Part model, mm, in its own coordinate system. Face numbers are marked on the shaded views. A direction names the side the tool comes from. Round coordinates to 2 decimals unless told otherwise and drop trailing zeros. Write each loop counter-clockwise with the first axis right and the second up, starting at its lowest first coordinate (ties: lowest second). Pieces come first, ordered by that corner, then holes. Notation, with made-up numbers: M 3.5,33.25 L 21.5,33.25 A29 cw 21.5,60.25 Z; hole C 72,45 d2. An arc over 180 degrees is marked long. One line per question, with ' | ' between items. Start each with the question number.
1) Saw through at C-C (x = -48). List the corners of the cut face in (y, z).
2) Wall check: probe 1 along Z at (x, y) = (-23, 23.5); probe 2 along Y at (x, z) = (32, 54.5); probe 3 along Y at (x, z) = (18.5, -50.5). Give the ranges that are in metal, low to high. Write a range as [from, to].
3) Saw through at A-A (x = 20). List the corners of the cut face in (y, z), plus the area to 3 significant figures.
4) Tool access for the marked faces 1, 2 and 3: list every direction of +Z, -Z, +X, -X, +Y, -Y with a clear straight run to the whole face (end or side of a thin tool).
5) Saw through at B-B (y = 6.25). List the corners of the cut face in (x, z), plus the area to 3 significant figures.
6) Saw through at D-D (z = -35.5). List the corners of the cut face in (x, y), plus the area to 3 significant figures.
7) Drop flat-ended pins along their axis: pin 1 Ø10 at (x, z) = (-9.5, 10.5) entering from -Y; pin 2 Ø12 at (x, y) = (-20.5, 15) entering from -Z; pin 3 Ø8 at (x, z) = (-27.5, 48) entering from -Y; pin 4 Ø16 at (x, z) = (-19.5, 4) entering from -Y. Give the stop position or say it passes through.
8) Mould opens along X. For the marked faces 4, 5 and 6 say: pulls with the +X half, pulls with the -X half, needs draft (parallel to the pull), parting line crosses it, or undercut.
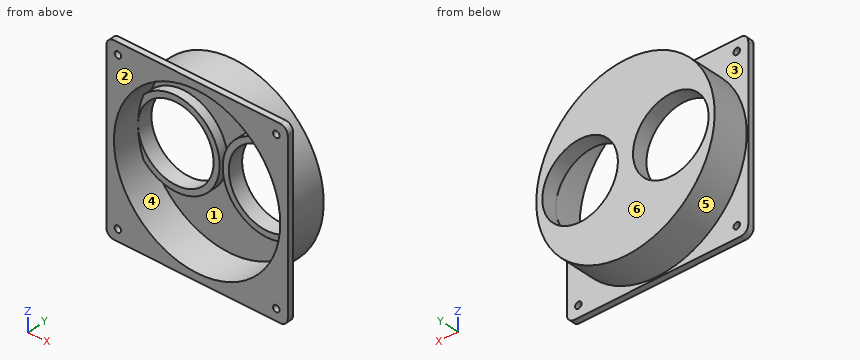
```python
from build123d import *

# Parameters (mm, degrees)
SKETCH1_W           = 120
SKETCH1_H           = 120
BOSS_EXTRUDE1_DEPTH = 4
FILLET1_R           = 5
SKETCH2_R           = 2.15
CUT_EXTRUDE1_DEPTH  = 4
SKETCH3_R           = 55
CUT_EXTRUDE2_DEPTH  = 4
BOSS_EXTRUDE2_START = 20
SKETCH5_R           = 59
SKETCH5_R_2         = 55
BOSS_EXTRUDE2_DEPTH = 20
BOSS_EXTRUDE3_START = 4
SKETCH6_R           = 59
BOSS_EXTRUDE3_DEPTH = 4
SKETCH7_R           = 25
CUT_EXTRUDE3_DEPTH  = 4
SKETCH8_R           = 29
SKETCH8_R_2         = 25
BOSS_EXTRUDE4_DEPTH = 6


with BuildPart() as part:
    # Sketch1 → Boss-Extrude1 (new body)
    with BuildSketch(Plane(origin=(0, 0, 0), x_dir=(1, 0, 0), z_dir=(0, 1, 0))):
        Rectangle(SKETCH1_W, SKETCH1_H)
    extrude(amount=BOSS_EXTRUDE1_DEPTH)

    # Fillet1
    fillet1_edges = [part.edges().sort_by_distance(p)[0] for p in [
        (60, 2, 60),
        (-60, 2, 60),
        (-60, 2, -60),
        (60, 2, -60),
    ]]
    fillet(fillet1_edges, radius=FILLET1_R)

    # Sketch2 → Cut-Extrude1 (cut)
    with BuildSketch(Plane(origin=(0, 4, 0), x_dir=(1, 0, 0), z_dir=(0, 1, 0))):
        with Locations(Location((-52.4, 52.4, 0), (0, 0, 270))):
            Circle(SKETCH2_R)
        with Locations(Location((52.4, 52.4, 0), (0, 0, 270))):
            Circle(SKETCH2_R)
        with Locations(Location((-52.4, -52.4, 0), (0, 0, 270))):
            Circle(SKETCH2_R)
        with Locations(Location((52.4, -52.4, 0), (0, 0, 270))):
            Circle(SKETCH2_R)
    extrude(amount=-CUT_EXTRUDE1_DEPTH, mode=Mode.SUBTRACT)

    # Sketch3 → Cut-Extrude2 (cut)
    with BuildSketch(Plane(origin=(0, 4, 0), x_dir=(1, 0, 0), z_dir=(0, 1, 0))):
        with Locations(Location((0, 0, 0), (0, 0, 270))):
            Circle(SKETCH3_R)
    extrude(amount=-CUT_EXTRUDE2_DEPTH, mode=Mode.SUBTRACT)

    # Sketch5 → Boss-Extrude2 (add)
    with BuildSketch(Plane(origin=(0, 4, 0), x_dir=(1, 0, 0), z_dir=(0, 1, 0)).offset(BOSS_EXTRUDE2_START)):
        with Locations(Location((0, 0, 0), (0, 0, 270))):
            Circle(SKETCH5_R)
        with Locations(Location((0, 0, 0), (0, 0, 270))):
            Circle(SKETCH5_R_2, mode=Mode.SUBTRACT)
    extrude(amount=-BOSS_EXTRUDE2_DEPTH)

    # Sketch6 → Boss-Extrude3 (add)
    with BuildSketch(Plane(origin=(0, 24, 0), x_dir=(1, 0, 0), z_dir=(0, 1, 0)).offset(BOSS_EXTRUDE3_START)):
        with Locations(Location((0, 0, 0), (0, 0, 270))):
            Circle(SKETCH6_R)
    extrude(amount=-BOSS_EXTRUDE3_DEPTH)

    # Sketch7 → Cut-Extrude3 (cut)
    with BuildSketch(Plane(origin=(0, 28, 0), x_dir=(1, 0, 0), z_dir=(0, 1, 0))):
        with Locations(Location((30, 0, 0), (0, 0, 270))):
            Circle(SKETCH7_R)
        with Locations(Location((-30, 0, 0), (0, 0, 270))):
            Circle(SKETCH7_R)
    extrude(amount=-CUT_EXTRUDE3_DEPTH, mode=Mode.SUBTRACT)

    # Sketch8 → Boss-Extrude4 (add)
    # profile 1 of 2: a face of its own
    with BuildSketch(Plane.XZ.offset(-24)):
        with Locations((30, 0)):
            Circle(SKETCH8_R)
        with Locations(Location((30, 0, 0), (0, 0, 90))):
            Circle(SKETCH8_R_2, mode=Mode.SUBTRACT)
    # profile 2 of 2: a face of its own
    with BuildSketch(Plane.XZ.offset(-24)):
        with Locations((-30, 0)):
            Circle(SKETCH8_R)
        with Locations(Location((-30, 0, 0), (0, 0, 90))):
            Circle(SKETCH8_R_2, mode=Mode.SUBTRACT)
    extrude(amount=BOSS_EXTRUDE4_DEPTH)


solid = part.part
```
Answer key:
1) outline: M 0,-60 L 4,-60 L 4,-34.31 L 28,-34.31 L 28,-17.35 L 18,-17.35 L 18,-22.74 L 24,-22.74 L 24,-26.85 L 0,-26.85 Z; M 0,26.85 L 24,26.85 L 24,22.74 L 18,22.74 L 18,17.35 L 28,17.35 L 28,34.31 L 4,34.31 L 4,60 L 0,60 Z
2) probe 1: z = [-54.33, -49.96], [-28.14, -24], [24, 28.14], [49.96, 54.33] | probe 2: y = [0, 4] | probe 3: y = [24, 28]
3) outline: M 0,-60 L 4,-60 L 4,-55.51 L 28,-55.51 L 28,-22.91 L 18,-22.91 L 18,-27.22 L 24,-27.22 L 24,-51.23 L 0,-51.23 Z; M 0,51.23 L 24,51.23 L 24,27.22 L 18,27.22 L 18,22.91 L 28,22.91 L 28,55.51 L 4,55.51 L 4,60 L 0,60 Z | area: 553 mm2
4) face 1: -Y | face 2: +Z, -Z, +X, -X, -Y | face 3: +Y
5) outline: C 0,0 d118; hole C 0,0 d110 | area: 1,430 mm2
6) outline: M -60,0 L -42.01,0 L -42.01,24 L 42.01,24 L 42.01,0 L 60,0 L 60,4 L 47.12,4 L 47.12,28 L -47.12,28 L -47.12,4 L -60,4 Z | area: 726 mm2
7) pin 1: stops at y = 18 | pin 2: stops at z = -57.19 | pin 3: stops at y = 0 | pin 4: passes through
8) face 4: undercut | face 5: parting line crosses it | face 6: needs draft
